Geometry: final body of the model. Coordinates: model frame, mm. A direction names the side the tool comes from. Round coordinates to 2 decimals unless told otherwise and drop trailing zeros. Write each loop counter-clockwise with the first axis right and the second up, starting at its lowest first coordinate (ties: lowest second). Pieces come first, ordered by that corner, then holes. Notation, with made-up numbers: (47.25, -1) -> (56.25, -1) arc R27 ccw to (56.25, 34) -> close; hole circle Ø2 at (77, 84.25). An arc over 180 degrees is marked (long way). One line per item, written item: value. Start each with the question number.
from build123d import *

# Parameters (mm, degrees)
SKETCH3_R           = 0.35052
BOSS_EXTRUDE1_DEPTH = 0.2032


with BuildPart() as part:
    # Sketch1 → Revolve1 (revolve)
    with BuildSketch(Plane(origin=(0, 0, 0), x_dir=(0, 0, -1), z_dir=(1, 0, 0))):
        Polygon((0, 0), (0, 2.9972), (15.0368, 2.9972), (15.0368, 1.5875), (15.4178, 1.5875), (15.4178, 0), align=None)
    revolve(axis=Axis((0, 0, -15.4178), (0, 0, 1)))

    # Sketch3 → Boss-Extrude1 (add)
    with BuildSketch(Plane(origin=(1.6256, 0, 0), x_dir=(0, 0, -1), z_dir=(1, 0, 0))):
        with BuildLine():
            Line((15.0368, 0.635), (15.0368, -0.635))
            Line((15.0368, -0.635), (15.6718, -0.635))
            ThreePointArc((15.6718, -0.635), (15.882828569, -0.543684888), (16.108651936, -0.50038))
            Line((16.108651936, -0.50038), (18.0086, -0.50038))
            ThreePointArc((18.0086, -0.50038), (18.237732209, 0), (18.0086, 0.50038))
            Line((18.0086, 0.50038), (16.108651936, 0.50038))
            ThreePointArc((16.108651936, 0.50038), (15.882828569, 0.543684888), (15.6718, 0.635))
            Line((15.6718, 0.635), (15.0368, 0.635))
        make_face()
        with Locations((17.5768, 0)):
            Circle(SKETCH3_R, mode=Mode.SUBTRACT)
    boss_extrude1 = extrude(amount=BOSS_EXTRUDE1_DEPTH)

    # Mirror1: Boss-Extrude1 across plane
    add(boss_extrude1.mirror(Plane(origin=(0, 0, 0), x_dir=(0, 0, 1), z_dir=(1, 0, 0))))


solid = part.part
(1) Section query A-A (y = 0). Count the separate pieces of the cut face and the enclosed holes in it, and give its area (3 significant figures).
(2) Set-up query: faces 1 (the face through (0, 0, 0)), 2 (the face through (0, 0, -15.418)). Return all of +Z, -Z, +X, -X, +Y, -Y with unobstructed straight access to the full face (end or side cutting, diameter ignored); none if empty.
(3) Pull-direction query (X, two-part tool) for faces 3 (the face through (-1.829, 0, -16)), 4 (the face through (1.829, 0, -16)), 5 (the face through (1.41, 0.73, -15.23)); classes: pulls with the +X half, pulls with the -X half, needs draft (parallel to the pull), parting line crosses it, or undercut.
(4) Section query B-B (x = 0). Output: boundary loops of the cut face in (y, z).
(5) Section query C-C (z = -8). Output: boundary loops of the cut face in (x, y).
(6) Line query: probe 1 along Z at (x, y) = (1.15, -0.3); probe 2 along Y at (x, z) = (0.15, -4.25); probe 3 along Z at (x, y) = (2.1, 2.1). Output: solid intervals per line, ascending.
(7) Section query D-D (y = -2.15). Output: boundary loops of the cut face in (x, z).
(8) Pin query (flat end, axial travel): pin 1 (0.6 mm diameter, centred on y = 0, z = -16, fed in from +X); pin 2 (1.4 mm diameter, centred on y = 0, z = -16, fed in from -X); pin 3 (1.5 mm diameter, centred on x = -1, z = -12, fed in from -Y). Return the tip coordinate at first contact, or that it passes through.
Results list:
1. separate pieces: 3
1. enclosed holes: 0
1. area: 92.4 mm^2
2. face 1: +Z, +X, -X, +Y, -Y
2. face 2: -Z, +Y, -Y
3. face 3: pulls with the -X half
3. face 4: pulls with the +X half
3. face 5: undercut
4. outline: (-3, -15.04) -> (-1.59, -15.04) -> (-1.59, -15.42) -> (1.59, -15.42) -> (1.59, -15.04) -> (3, -15.04) -> (3, 0) -> (-3, 0) -> close
5. outline: circle Ø5.99 at (0, 0)
6. probe 1: z = -15.42 to 0
6. probe 2: y = -2.99 to 2.99
6. probe 3: z = -15.04 to 0
7. outline: (-2.09, -15.04) -> (2.09, -15.04) -> (2.09, 0) -> (-2.09, 0) -> close
8. pin 1: stops at x = 1.83
8. pin 2: stops at x = -1.83
8. pin 3: stops at y = -2.99
